The drawing under review shows one solid part. Ordinate dimensions are in mm from its lowest x, y, z. A direction names the side the tool comes from. Coordinates: 2 decimals unless noted, no trailing zeros. Write each loop counter-clockwise with the first axis right and the second up, starting at its lowest first coordinate (ties: lowest second). Pieces come first, ordered by that corner, then holes.
1) For the marked faces 1 and 2, list the 3-axis set-ups (+Z, -Z, +X, -X, +Y, -Y) from which the entire face can be reached by the end or side of a thin tool; tool diameter is ignored.
2) We need section A-A on z = 57.5. Write out the cut boundary in (x, y), then the cut area to 3 significant figures.
3) Mouldability with a two-part tool opening along Y and no side actions: class the marked faces 3, 4, 5 and 6 as pulls with the +Y half, pulls with the -Y half, needs draft (parallel to the pull), parting line crosses it, or undercut.
4) We need section C-C on y = 264.5. Write out the cut boundary in (x, z), then the cut area to 3 significant figures.
5) To check wall thickness, follow line 1 along Y through (x, z) = (581.5, 80.5); line 2 along Z through (x, y) = (772, 577). State the ranges of each line that lie inside material, in increasing order.
6) We need section B-B on x = 1012. Write out the cut boundary in (y, z).
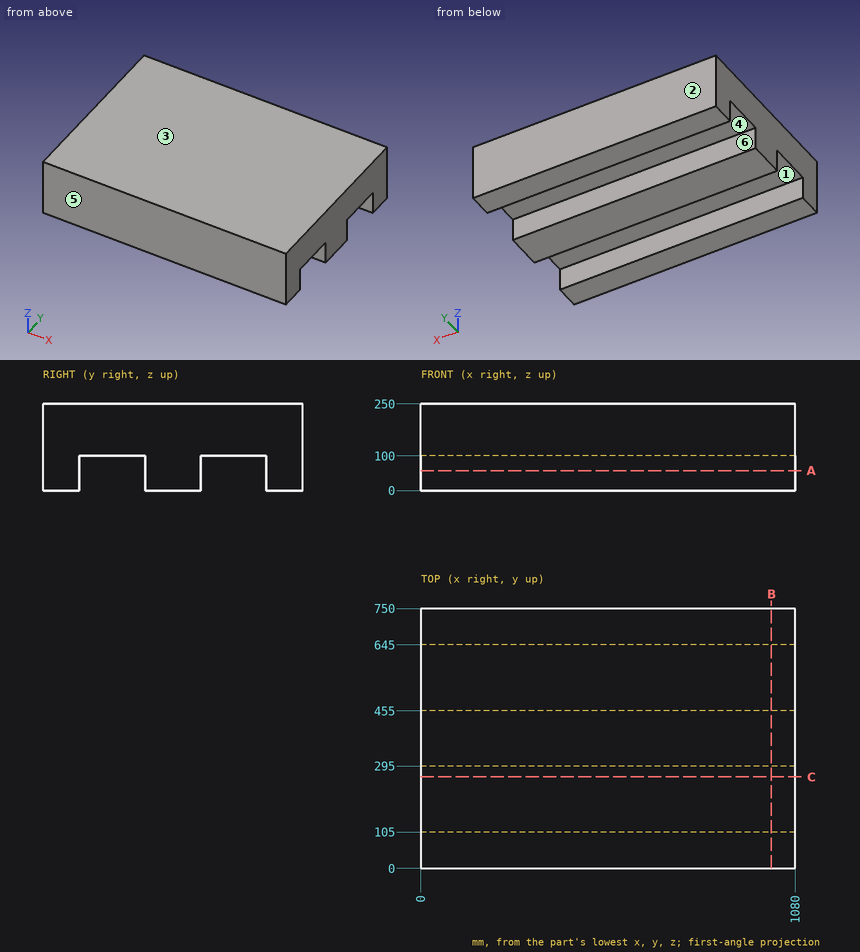
Result:
1. face 1: -Z, +X, -X
1. face 2: +Z, -Z, +X, -X, +Y
2. outline: (0, 0) - (1080, 0) - (1080, 105) - (0, 105) - close; (0, 295) - (1080, 295) - (1080, 455) - (0, 455) - close; (0, 645) - (1080, 645) - (1080, 750) - (0, 750) - close
2. area: 400,000 mm2
3. face 3: needs draft
3. face 4: undercut
3. face 5: pulls with the -Y half
3. face 6: undercut
4. outline: (0, 100) - (1080, 100) - (1080, 250) - (0, 250) - close
4. area: 162,000 mm2
5. line 1: y = 0 to 105, 295 to 455, 645 to 750
5. line 2: z = 100 to 250
6. outline: (0, 0) - (105, 0) - (105, 100) - (295, 100) - (295, 0) - (455, 0) - (455, 100) - (645, 100) - (645, 0) - (750, 0) - (750, 250) - (0, 250) - close
